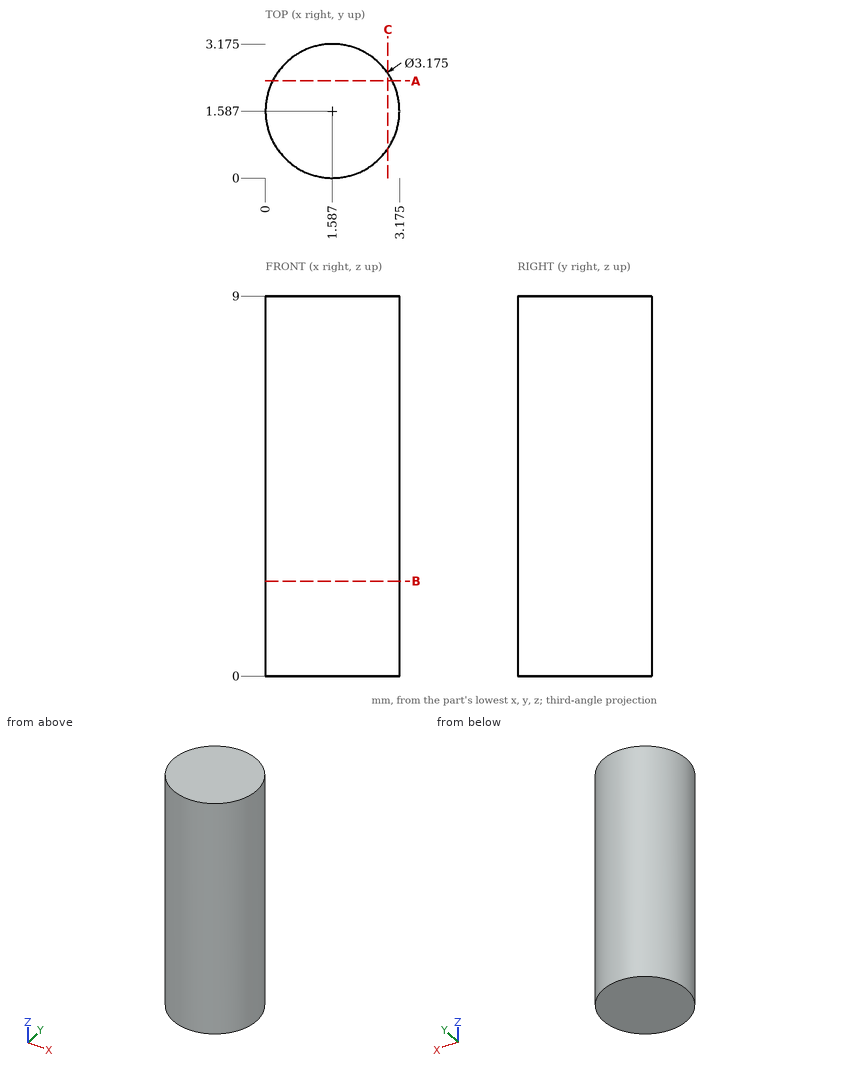
Could you check a few things on this drawing? It's one solid part, dimensions in mm from its lowest x, y, z. Give positions to 0.01 mm unless a question says otherwise; leave off trailing zeros. Write each loop counter-clockwise with the first axis right and the second up, starting at its lowest first coordinate (ties: lowest second). Pieces come first, ordered by that corner, then holes. Notation, with made-up numbers: (2.25, 67) -> (56.25, 67) arc R31 cw to (56.25, 99) -> close; hole circle Ø9 at (27, 48.5). An arc over 180 degrees is marked (long way). Write item = value, one per line.
(1) Suppose I cut it at C-C on x = 2.9. Write out the boundary of the cut face in (y, z) (1 decimal), then the cut area to 3 significant figures.
Worked out:
outline = (0.7, 0) -> (2.5, 0) -> (2.5, 9) -> (0.7, 9) -> close
area = 16.1 mm^2
(2) I'm going to push a flat-ended pin straight in: P1, Ø1, axis at x = 2, z = 7.5, coming from the +Y side (1 decimal). Where does the tip first touch, or does it pass through?
Worked out:
P1 = 3.2
(3) I need wall thicknesses on probe 1 along X at (y, z) = (0.6, 8.75) (1 decimal); probe 2 along X at (y, z) = (1.15, 5.5) (1 decimal); probe 3 along Y at (x, z) = (1.9, 8.5) (1 decimal). Which ranges of each line are inside material? Lowest first, please. Write a range as from..to.
Worked out:
probe_1 = 0.3..2.8
probe_2 = 0.1..3.1
probe_3 = 0..3.1
(4) Suppose I cut it at A-A on y = 2.3. Write out the boundary of the cut face in (x, z).
Worked out:
outline = (0.17, 0) -> (3.01, 0) -> (3.01, 9) -> (0.17, 9) -> close
(5) Suppose I cut it at B-B on z = 2.25. Write out the boundary of the cut face in (x, y) (1 decimal).
Worked out:
outline = circle Ø3.2 at (1.6, 1.6)
